from build123d import *

# Parameters (mm, degrees)
ESQUISSE1_R        = 85
BOSS_EXTRU_1_DEPTH = 150
ESQUISSE2_W        = 180
ESQUISSE2_H        = 180
BOSS_EXTRU_2_DEPTH = 20
CONG_1_R           = 5
CONG_2_R           = 5
CONG_3_R           = 5
CONG_4_R           = 5
CONG_5_R           = 5
ESQUISSE4_R        = 15
BOSS_EXTRU_3_DEPTH = 600


with BuildPart() as part:
    # Esquisse1 → Boss.-Extru.1 (new body)
    with BuildSketch(Plane.XY):
        Circle(ESQUISSE1_R)
    extrude(amount=BOSS_EXTRU_1_DEPTH)

    # Esquisse2 → Boss.-Extru.2 (add)
    with BuildSketch(Plane.XY.offset(150)):
        Rectangle(ESQUISSE2_W, ESQUISSE2_H)
    extrude(amount=BOSS_EXTRU_2_DEPTH)

    # Congé1
    cong_1_edges = [part.edges().sort_by_distance(p)[0] for p in [
        (-85, 0, 150),
    ]]
    fillet(cong_1_edges, radius=CONG_1_R - 0.0001)  # a hair under: the kernel refuses the full size

    # Congé2
    cong_2_edges = [part.edges().sort_by_distance(p)[0] for p in [
        (-90, 90, 160),
    ]]
    fillet(cong_2_edges, radius=CONG_2_R)

    # Congé3
    cong_3_edges = [part.edges().sort_by_distance(p)[0] for p in [
        (-90, -90, 160),
    ]]
    fillet(cong_3_edges, radius=CONG_3_R)

    # Congé4
    cong_4_edges = [part.edges().sort_by_distance(p)[0] for p in [
        (90, 90, 160),
    ]]
    fillet(cong_4_edges, radius=CONG_4_R)

    # Congé5
    cong_5_edges = [part.edges().sort_by_distance(p)[0] for p in [
        (90, -90, 160),
    ]]
    fillet(cong_5_edges, radius=CONG_5_R)

    # Esquisse4 → Boss.-Extru.3 (add)
    with BuildSketch(Plane(origin=(0, 0, 0), x_dir=(0, 0, -1), z_dir=(1, 0, 0))):
        with Locations(Location((-135, 0, 0), (0, 0, 180))):
            Circle(ESQUISSE4_R)
    extrude(amount=BOSS_EXTRU_3_DEPTH)


solid = part.part
Here's how the part is built. I have some questions about the finished solid (model axes, mm). A direction names the side the tool comes from. Give positions to 0.01 mm unless a question says otherwise; leave off trailing zeros. Order: outer loops, then holes, each group sorted by start corner. A loop starts at its lowest first (then second) coordinate and runs counter-clockwise, first axis right, second up. Notation, with made-up numbers: (-13, 69) -> (0, 69) arc R19 cw to (0, 75) -> close; hole circle Ø1 at (16.25, 59). An arc over 180 degrees is marked (long way). One line per item, written item: value. Start each with the question number.
1. Will these pins go through, and if not, where does the flat tip stop? pin 1 Ø2 at (x, z) = (-15, 24) entering from +Y; pin 2 Ø6 at (y, z) = (20.5, 158.5) entering from +X; pin 3 Ø2 at (x, y) = (449, -14) entering from +Z.
2. Imagine slicing it at C-C, the plane x = 287.5. List the corners of the cut face in (y, z) for me.
3. I need wall thicknesses on probe 1 along X at (y, z) = (13, 157); probe 2 along Z at (x, y) = (-21.5, 83.5); probe 3 along Y at (x, z) = (49, 51.5). Which ranges of each line are inside material? Lowest first, please. Write a range as from..to.
4. For faces 1 (the face through (-67.453, -51.721, 71.485)), 2 (the face through (-1, 1, 170)), 3 (the face through (338.218, -0.66, 120.015)), which set-ups out of +Z, -Z, +X, -X, +Y, -Y let a thin tool reach every point of the face, with its end or its side?
5. Imagine slicing it at B-B, the plane z = 135. List the corners of the cut face in (x, y) for me.
Values follow:
1. pin 1: stops at y = 83.84
1. pin 2: stops at x = 90
1. pin 3: stops at z = 142.48
2. outline: circle Ø30 at (0, 135)
3. probe 1: x = -90..90
3. probe 2: z = 148.28..170
3. probe 3: y = -69.46..69.46
4. face 1: -Z
4. face 2: +Z, +X, -X, +Y, -Y
4. face 3: +X
5. outline: (83.67, -15) -> (600, -15) -> (600, 15) -> (83.67, 15) arc R85 ccw (long way) to start
